The listing builds one solid part. Answer for the finished solid, in the listing's coordinates (mm). A direction names the side the tool comes from. Coordinates: 2 decimals unless noted, no trailing zeros. Order: outer loops, then holes, each group sorted by start corner. A loop starts at its lowest first (then second) coordinate and runs counter-clockwise, first axis right, second up. Notation, with made-up numbers: (80, 27.5) - (120, 27.5) arc R22 ccw to (120, 48.5) - close; hole circle Ø5 at (25.25, 87.25). An arc over 180 degrees is marked (long way). Use a Markdown table: item, result. Add a question column.
Item 1: For faces 1 (the flat face through (4, 2, -43.18)), 2 (the cylindrical face through (48.3, 2.2, -49.4)), 3 (the cylindrical face through (19.512, 30.257, -49.441)), 4 (the cylindrical face through (49.742, -23.347, -49.441)), determine the directions among +Z, -Z, +X, -X, +Y, -Y from which every point of the face is accessible in a straight line to the end or side of a thin tool.
Item 2: The mould has two halves that part along X. Classify faces 5 (the flat face through (4, -15, -55.88)), 6 (the conical face through (1.614, 6.603, -53.463)), 7 (the cylindrical face through (8.816, -6.643, -21.288)): released by +X, released by -X, zero draft, split by the parting line, or undercut.
Item 3: The part is cut by section A-A, the plane y = 35.5. State how many separate pieces and enclosed holes the cut face has, then the cut area to 3 significant figures.
Item 4: The part is cut by section B-B, the plane z = -5.5. Give the vertices of the cut face in (x, y) (3 decimals), then the cut area to 3 significant figures.
Item 5: Find the intervals of material crossed by line 1 along Z through (x, y) = (22, -12); line 2 along Z through (x, y) = (6, -14); line 3 along X through (y, z) = (8.5, -33), in increasing order.
Item 6: Flat-ended cylindrical pins translate along their axes: P1, Ø6, axis at y = 12, z = -44, coming from the -X side (3 decimals); P2, Ø12, axis at y = 27.5, z = -2, coming from the +X side; P3, Ø8, axis at x = -5.5, y = -23.54, coming from the -Z side. Find the tip coordinate at first contact, or state that the pin passes through.
from build123d import *

# Parameters (mm, degrees)
SKETCH1_R           = 4.445
BOSS_EXTRUDE1_DEPTH = 10.16
FILLET1_R           = 12.7
SKETCH2_R           = 13.97
BOSS_EXTRUDE2_DEPTH = 43.18
SKETCH4_R           = 4.445
BOSS_EXTRUDE3_DEPTH = 12.7
SKETCH5_R           = 9.525
CUT_EXTRUDE2_DEPTH  = 109.223551539
SKETCH6_R           = 19.05
CUT_EXTRUDE3_DEPTH  = 2.54
CHAMFER1_SIZE       = 2.54
FILLET2_R           = 2.54


with BuildPart() as part:
    # Sketch1 → Boss-Extrude1 (new body)
    with BuildSketch(Plane.XY):
        Polygon((10.696130127, -43.269340837), (-25.224894357, -7.348316353), (-34.430434771, 1.857224061), (-25.224894357, 11.062764475), (10.696130127, 46.98378896), (19.901670541, 56.189329374), (29.107210955, 46.98378896), (65.02823544, 11.062764475), (74.233775854, 1.857224061), (65.02823544, -7.348316353), (29.107210955, -43.269340837), (19.901670541, -52.474881251), align=None)
        with Locations((-16.019353943, 1.857224061)):
            Circle(SKETCH1_R, mode=Mode.SUBTRACT)
        with Locations((19.901670541, 37.778248545)):
            Circle(SKETCH1_R, mode=Mode.SUBTRACT)
        with Locations((19.901670541, -34.063800423)):
            Circle(SKETCH1_R, mode=Mode.SUBTRACT)
        with Locations((55.822695025, 1.857224061)):
            Circle(SKETCH1_R, mode=Mode.SUBTRACT)
    extrude(amount=BOSS_EXTRUDE1_DEPTH)

    # Fillet1
    fillet1_edges = [part.edges().sort_by_distance(p)[0] for p in [
        (-34.430434771, 1.857224061, 5.08),
        (19.901670541, 56.189329374, 5.08),
        (74.233775854, 1.857224061, 5.08),
        (19.901670541, -52.474881251, 5.08),
    ]]
    fillet(fillet1_edges, radius=FILLET1_R)

    # Sketch2 → Boss-Extrude2 (add)
    with BuildSketch(Plane.XY):
        with Locations((19.901670541, 1.857224061)):
            Circle(SKETCH2_R)
    extrude(amount=-BOSS_EXTRUDE2_DEPTH)

    # Sketch4 → Boss-Extrude3 (add)
    with BuildSketch(Plane(origin=(0, 0, -43.18), x_dir=(-1, 0, 0), z_dir=(0, 0, -1))):
        with BuildLine():
            ThreePointArc((-45.301670541, 39.957224061), (-54.281926662, 36.237480182), (-58.001670541, 27.257224061))
            ThreePointArc((-58.001670541, 27.257224061), (-48.299733855, 1.857224061), (-58.001670541, -23.542775939))
            ThreePointArc((-58.001670541, -23.542775939), (-54.281926662, -32.52303206), (-45.301670541, -36.242775939))
            ThreePointArc((-45.301670541, -36.242775939), (-19.901670541, -26.540839253), (5.498329459, -36.242775939))
            ThreePointArc((5.498329459, -36.242775939), (14.47858558, -32.52303206), (18.198329459, -23.542775939))
            ThreePointArc((18.198329459, -23.542775939), (8.496392773, 1.857224061), (18.198329459, 27.257224061))
            ThreePointArc((18.198329459, 27.257224061), (14.47858558, 36.237480182), (5.498329459, 39.957224061))
            ThreePointArc((5.498329459, 39.957224061), (-19.901670541, 30.255287375), (-45.301670541, 39.957224061))
        make_face()
        with Locations((-45.301670541, 27.257224061)):
            Circle(SKETCH4_R, mode=Mode.SUBTRACT)
        with Locations((5.498329459, 27.257224061)):
            Circle(SKETCH4_R, mode=Mode.SUBTRACT)
        with Locations((5.498329459, -23.542775939)):
            Circle(SKETCH4_R, mode=Mode.SUBTRACT)
        with Locations((-45.301670541, -23.542775939)):
            Circle(SKETCH4_R, mode=Mode.SUBTRACT)
    extrude(amount=BOSS_EXTRUDE3_DEPTH)

    # Sketch5 → Cut-Extrude2 (cut, through all)
    with BuildSketch(Plane(origin=(0, 0, -55.88), x_dir=(-1, 0, 0), z_dir=(0, 0, -1))):
        with Locations((-19.901670541, 0.843392699)):
            Circle(SKETCH5_R)
    extrude(amount=-CUT_EXTRUDE2_DEPTH, mode=Mode.SUBTRACT)

    # Sketch6 → Cut-Extrude3 (cut)
    with BuildSketch(Plane(origin=(0, 0, -55.88), x_dir=(-1, 0, 0), z_dir=(0, 0, -1))):
        with Locations((-19.901670541, 0.843392699)):
            Circle(SKETCH6_R)
    extrude(amount=-CUT_EXTRUDE3_DEPTH, mode=Mode.SUBTRACT)

    # Chamfer1
    chamfer1_edges = [part.edges().sort_by_distance(p)[0] for p in [
        (38.951670541, 0.843392699, -55.88),
    ]]
    chamfer(chamfer1_edges, length=CHAMFER1_SIZE - 0.0001)  # a hair under: the kernel refuses the full size

    # Fillet2
    fillet2_edges = [part.edges().sort_by_distance(p)[0] for p in [
        (47.067723198, -25.308828595, 0),
        (-7.264382115, -25.308828595, 0),
        (-7.264382115, 29.023276718, 0),
        (47.067723198, 29.023276718, 0),
        (19.901670541, 50.928817132, 0),
        (-29.169922529, 1.857224061, 0),
        (68.973263612, 1.857224061, 0),
        (19.901670541, -47.214369009, 0),
    ]]
    fillet(fillet2_edges, radius=FILLET2_R)


solid = part.part
Solution:
| question | item | result |
|---|---|---|
| 1 | face 1 | none |
| 1 | face 2 | -Z, +X |
| 1 | face 3 | -Z, +Y |
| 1 | face 4 | -Z |
| 2 | face 5 | zero draft |
| 2 | face 6 | undercut |
| 2 | face 7 | split by the parting line |
| 3 | separate pieces | 4 |
| 3 | enclosed holes | 0 |
| 3 | area | 740 mm2 |
| 4 | outline | circle Ø27.94 at (19.902, 1.857); hole circle Ø19.05 at (19.902, 0.843) |
| 4 | area | 328 mm2 |
| 5 | line 1 | z = -53.34 to -43.18, 0 to 10.16 |
| 5 | line 2 | z = -54.63 to -43.18, 0 to 10.16 |
| 5 | line 3 | x = 7.61 to 14.24, 25.57 to 32.19 |
| 6 | P1 | stops at x = -10.835 |
| 6 | P2 | stops at x = 53.15 |
| 6 | P3 | stops at z = 0 |
